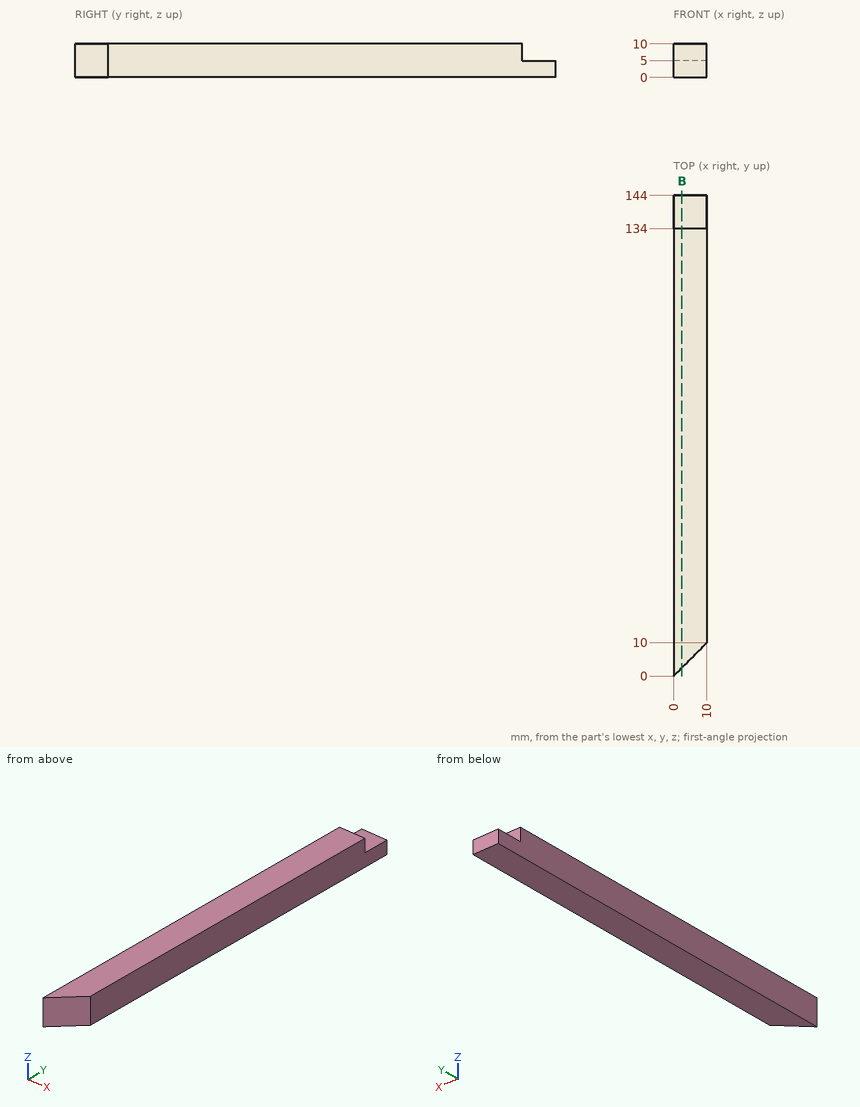
Drawing for the job (mm, zero at the part's lowest x, y, z). Give positions to 0.01 mm unless a question says otherwise; leave off trailing zeros. Order: outer loops, then holes, each group sorted by start corner. A loop starts at its lowest first (then second) coordinate and runs counter-clockwise, first axis right, second up. Notation, with made-up numbers: M 73.5,-8 L 109.5,-8 A29 cw 109.5,16 Z; hole C 4,42 d9. An arc over 180 degrees is marked long. Use a Markdown table: item, result. Add a question column.
(1) Drop flat-ended pins along their axis: P1, Ø6, axis at x = 5.5, z = 9, coming from the +Y side; P2, Ø6, axis at x = 4.5, z = 8.5, coming from the -Y side; P3, Ø1, axis at x = 2.5, z = 2, coming from the -Y side. Give the stop position or say it passes through.
(2) Probe line 1 along Y through (x, z) = (3.5, 2.25); line 2 along Y through (x, z) = (2.25, 6.5). List the from-to ranges inside material, lowest first. Write a range as [from, to].
(3) Saw through at B-B, the plane x = 2.5. Give the cut face in (y, z), and give its area (4 significant figures).
Answer key:
| question | item | result |
|---|---|---|
| 1 | P1 | y = 134 |
| 1 | P2 | y = 1.5 |
| 1 | P3 | y = 2 |
| 2 | line 1 | [3.5, 144] |
| 2 | line 2 | [2.25, 134] |
| 3 | outline | M 2.5,0 L 144,0 L 144,5 L 134,5 L 134,10 L 2.5,10 Z |
| 3 | area | 1,365 mm^2 |
